The model under review builds one solid part; all positions refer to its coordinate system, in mm. Face numbers are marked on the shaded views. A direction names the side the tool comes from. Round coordinates to 2 decimals unless told otherwise and drop trailing zeros. Order: outer loops, then holes, each group sorted by start corner. A loop starts at its lowest first (then second) coordinate and runs counter-clockwise, first axis right, second up. Notation, with made-up numbers: (60, 54) - (83, 54) arc R23 cw to (83, 68) - close; hole circle Ø8 at (-21.75, 43.5). An arc over 180 degrees is marked (long way). One line per question, with ' | ' between items. Start each with the question number.
Item 1: Add section B-B on x = 9.5. State the section outline as (y, z) points.
Item 2: Draft analysis for pull direction X (two halves, no side actions). For the marked faces 3, 4 and 5, state which applies: +X half, -X half, draft (parallel to the pull), parting line (faces both ways), or undercut.
Item 3: For L1, parallel to X at y = 2.4, z = 2.6; L2, parallel to X at y = 3.2, z = 4.4; L3, parallel to Y at x = 10, z = 2.1, list the stretches that pass through material, from the lowest coordinate up. Write a range as [from, to].
Item 4: Add section A-A on z = 4.4. State the section outline as (x, y) points.
Item 5: Insertion check: pin 1 Ø3 at (x, z) = (23, 5) entering from +Y; pin 2 Ø3 at (x, z) = (31.5, 3) entering from +Y. Each pin has a flat end and moves straight along its axis. Give the tip position at first contact, or say it passes through.
Item 6: Add section C-C on z = 2.05. State the section outline as (x, y) points.
Item 7: Add section D-D on x = 25. State the section outline as (y, z) points, and give its area (3 significant figures).
Item 8: Tool access review of the marked faces 1 and 2: name each direction out of +Z, -Z, +X, -X, +Y, -Y from which nothing blocks a thin tool from reaching the whole face with its end or side.
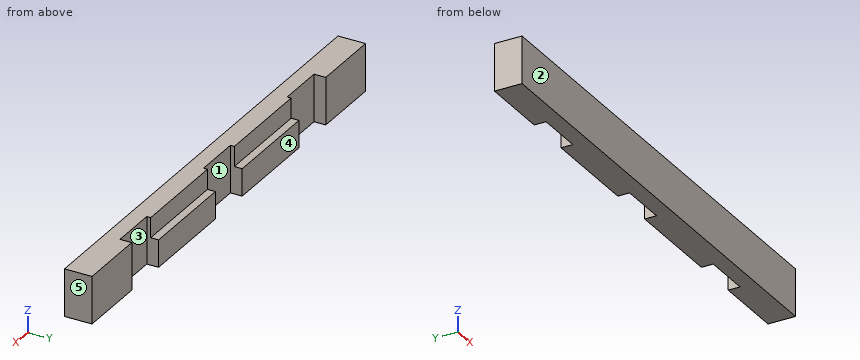
Autodesk Inventor part; units mm, degrees
ref_plane "YZ Plane" through (0, 0, 0) normal (1, 0, 0) x (0, 1, 0)
ref_plane "XZ Plane" through (0, 0, 0) normal (0, 1, 0) x (-1, 0, 0)
ref_plane "XY Plane" through (0, 0, 0) normal (0, 0, 1) x (1, 0, 0)
sketch "Sketch1" plane through (0, 0, 0) normal (0, 0, 1) x (1, 0, 0)
  line L0 (0, 0) -> (61.18, 0)
  line L1 (61.18, 0) -> (61.18, 2)
  line L2 (61.18, 2) -> (0, 2)
  line L3 (0, 2) -> (0, 0)
  line L4 (14.89, 2) -> (27.59, 2)
  line L5 (27.59, 2) -> (27.59, 3.5)
  line L6 (27.59, 3.5) -> (14.89, 3.5)
  line L7 (14.89, 3.5) -> (14.89, 2)
  line L8 (33.59, 2) -> (46.29, 2)
  line L9 (46.29, 2) -> (46.29, 3.5)
  line L10 (46.29, 3.5) -> (33.59, 3.5)
  line L11 (33.59, 3.5) -> (33.59, 2)
  line L12 (8.89, 2) -> (0, 2)
  line L13 (0, 2) -> (0, 3.5)
  line L14 (0, 3.5) -> (8.89, 3.5)
  line L15 (8.89, 3.5) -> (8.89, 2)
  line L16 (52.29, 2) -> (61.18, 2)
  line L17 (61.18, 2) -> (61.18, 3.5)
  line L18 (61.18, 3.5) -> (52.29, 3.5)
  line L19 (52.29, 3.5) -> (52.29, 2)
  dimension "d0" = 6
  dimension "d1" = 2
  dimension "d2" = 1.5
  dimension "d3" = 6
  dimension "d4" = 6
  dimension "d5" = 12.7
  dimension "d6" = 8.89
  dimension "d7" = 8.89
extrude "Extrusion1" add sketch "Sketch1" along normal blind 6
sketch "Sketch2" plane through (14.89, 3.5, 0) normal (0, 1, 0) x (1, 0, 0)
  line L0 (31.4, 0) -> (18.7, 0)
  line L1 (18.7, 0) -> (18.7, -6)
  line L2 (31.4, -6) -> (18.7, -6)
  line L3 (31.4, 0) -> (31.4, -6)
  line L4 (12.7, 0) -> (0, 0)
  line L5 (0, 0) -> (0, -6)
  line L6 (12.7, -6) -> (0, -6)
  line L7 (12.7, 0) -> (12.7, -6)
  line L8 (-14.89, -6) -> (46.29, -6)
  line L9 (18.7, -6) -> (31.4, -6)
  line L10 (31.4, -6) -> (31.4, -3.46)
  line L11 (31.4, -3.46) -> (18.7, -3.46)
  line L12 (18.7, -3.46) -> (18.7, -6)
  line L13 (12.7, 0) -> (12.7, -6)
  line L14 (0, -6) -> (12.7, -6)
  line L15 (12.7, -6) -> (12.7, -3.46)
  line L16 (12.7, -3.46) -> (0, -3.46)
  line L17 (0, -3.46) -> (0, -6)
  point P0 (-14.89, 0)
  point P1 (0, -3.46)
  dimension "d14" = 2.54
extrude "Extrusion2" cut sketch "Sketch2" against normal blind 1 contours L6 L5 L16 L7 | L3 L2 L1 L11
properties part number "Button Support"
Determined:
1) outline: (0, 0) - (2, 0) - (2, 6) - (0, 6) - close
2) face 3: undercut | face 4: draft | face 5: +X half
3) L1: [0, 8.89], [14.89, 27.59], [33.59, 46.29], [52.29, 61.18] | L2: [0, 8.89], [52.29, 61.18] | L3: [0, 2]
4) outline: (0, 0) - (61.18, 0) - (61.18, 3.5) - (52.29, 3.5) - (52.29, 2) - (46.29, 2) - (46.29, 2.5) - (33.59, 2.5) - (33.59, 2) - (27.59, 2) - (27.59, 2.5) - (14.89, 2.5) - (14.89, 2) - (8.89, 2) - (8.89, 3.5) - (0, 3.5) - close
5) pin 1: y = 2.5 | pin 2: y = 2
6) outline: (0, 0) - (61.18, 0) - (61.18, 3.5) - (52.29, 3.5) - (52.29, 2) - (46.29, 2) - (46.29, 3.5) - (33.59, 3.5) - (33.59, 2) - (27.59, 2) - (27.59, 3.5) - (14.89, 3.5) - (14.89, 2) - (8.89, 2) - (8.89, 3.5) - (0, 3.5) - close
7) outline: (0, 0) - (3.5, 0) - (3.5, 3.46) - (2.5, 3.46) - (2.5, 6) - (0, 6) - close | area: 18.5 mm2
8) face 1: +Z, -Z, +Y | face 2: +Z, -Z, +X, -X, -Y
